Design review of the part built by this model. Coordinates are the model's own, in mm. Face numbers are marked on the shaded views. Give positions to 0.01 mm unless a question says otherwise; leave off trailing zeros. Write each loop counter-clockwise with the first axis right and the second up, starting at its lowest first coordinate (ties: lowest second). Pieces come first, ordered by that corner, then holes. Notation, with made-up numbers: (15, -38.5) -> (32, -38.5) arc R26 cw to (32, -16.5) -> close; hole circle Ø5 at (74, 62.5). An arc over 180 degrees is marked (long way). Use CSV: the item, a comma, the result in double quotes.
```python
from build123d import *

# Parameters (mm, degrees)
F1_DEPTH = 18
F3_DEPTH = 6
F4_R     = 5
F5_DEPTH = 12
F6_W     = 10
F6_H     = 6
F7_DEPTH = 60


with BuildPart() as f1:
    # F0 (on Top) → F1 (new body)
    with BuildSketch(Plane.XY):
        Polygon((-35.3553390593, 35.3553390593), (0, 0), (25, 0), (25, 120.7106781187), (0, 120.7106781187), (-35.3553390593, 85.3553390593), align=None)
        Polygon((25, 120.7106781187), (25, 0), (50, 0), (85.3553390593, 35.3553390593), (85.3553390593, 85.3553390593), (50, 120.7106781187), align=None)
    extrude(amount=F1_DEPTH)

    # F2 (on face) → F3 (join)
    with BuildSketch(Plane.XY.offset(18)):
        Polygon((-35.3553390593, 85.3553390593), (-35.3553390593, 35.3553390593), (0, 0), (50, 0), (85.3553390593, 35.3553390593), (85.3553390593, 85.3553390593), (50, 120.7106781187), (0, 120.7106781187), align=None)
        Polygon((2.0710678119, 5), (-30.3553390593, 37.4264068712), (-30.3553390593, 83.2842712475), (2.0710678119, 115.7106781187), (47.9289321881, 115.7106781187), (80.3553390593, 83.2842712475), (80.3553390593, 37.4264068712), (47.9289321881, 5), align=None, mode=Mode.SUBTRACT)
        Polygon((-25.1553390593, 81.1303607231), (-25.1553390593, 39.5803173955), (4.2249783362, 10.2), (45.7750216638, 10.2), (75.1553390593, 39.5803173955), (75.1553390593, 81.1303607231), (45.7750216638, 110.5106781187), (4.2249783362, 110.5106781187), align=None)
    extrude(amount=F3_DEPTH)

    # F4 (on face) → F5 (cut)
    with BuildSketch(Plane.XY.offset(24)):
        with Locations((25, 60.3553390593)):
            Circle(F4_R)
    extrude(amount=-F5_DEPTH, mode=Mode.SUBTRACT)

    # F6 (on face) → F7 (cut)
    with BuildSketch(Plane(origin=(85.3553390593, 85.3553390593, 0), x_dir=(-0.7071067812, 0.7071067812, 0), z_dir=(0.7071067812, 0.7071067812, 0))):
        with Locations((25, 15)):
            Rectangle(F6_W, F6_H)
    extrude(amount=-F7_DEPTH, mode=Mode.SUBTRACT)


solid = f1.part
```
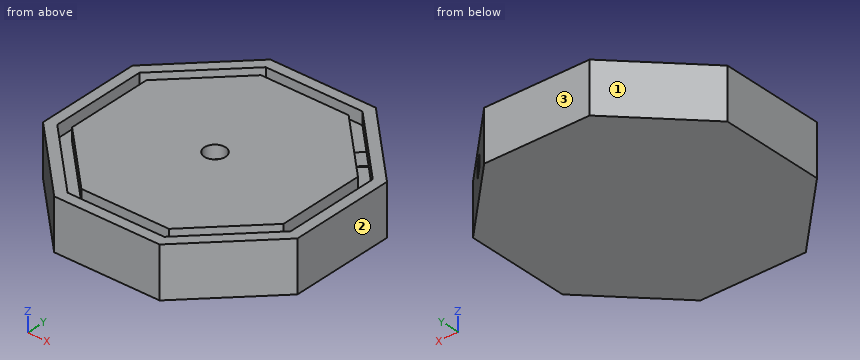
(1) Take a section at B-B (z = 6.25). Write out the cut boundary in (x, y), then the cut area to 3 significant figures.
Established:
outline,"(-35.36, 35.36) -> (0, 0) -> (50, 0) -> (85.36, 35.36) -> (85.36, 85.36) -> (50, 120.71) -> (0, 120.71) -> (-35.36, 85.36) -> close"
area,"12,100 mm2"
(2) Clearance check with flat-ended pins moving along their axes: pin 1 (10 mm diameter, centred on y = 13.5, z = 16, fed in from -X); pin 2 (10 mm diameter, centred on y = 27.5, z = 7.5, fed in from -X); pin 3 (1 mm diameter, centred on x = 52, z = 8, fed in from +Y). State where each tip first meets the part, or that it passes through.
Established:
pin 1,"stops at x = -18.5"
pin 2,"stops at x = -32.5"
pin 3,"stops at y = 119.21"
(3) Take a section at C-C (y = 33). Write out the cut boundary in (x, z).
Established:
outline,"(-33, 0) -> (83, 0) -> (83, 24) -> (75.93, 24) -> (75.93, 18) -> (68.58, 18) -> (68.58, 24) -> (-18.58, 24) -> (-18.58, 18) -> (-25.93, 18) -> (-25.93, 24) -> (-33, 24) -> close"
(4) For line 1 along Y through (x, z) = (25, 21.5); line 2 along Y through (x, z) = (25, 16.25); line 3 along Z through (x, y) = (39, 71), list the stretches that pass through material, from the lowest coordinate up. Write a range as [from, to].
Established:
line 1,"y = [0, 5], [10.2, 55.36], [65.36, 110.51], [115.71, 120.71]"
line 2,"y = [0, 55.36], [67.43, 120.71]"
line 3,"z = [0, 12], [18, 24]"
(5) Take a section at A-A (x = 15.5). Write out the cut boundary in (y, z).
Established:
outline,"(0, 0) -> (120.71, 0) -> (120.71, 24) -> (115.71, 24) -> (115.71, 18) -> (110.51, 18) -> (110.51, 24) -> (10.2, 24) -> (10.2, 18) -> (5, 18) -> (5, 24) -> (0, 24) -> close"
(6) Mouldability with a two-part tool opening along X and no side actions: class the marked faces 1, 2 and 3 as +X half, -X half, draft (parallel to the pull), parting line (faces both ways), or undercut.
Established:
face 1,"-X half"
face 2,"+X half"
face 3,"draft"
